Can you work these out from the model? Positions are in its coordinate system, mm. A direction names the side the tool comes from. Coordinates: 2 decimals unless noted, no trailing zeros. Loops run counter-clockwise (first coordinate to the right, second up) from the corner with the lowest first, then second, coordinate; pieces in that order, holes last. Notation, with made-up numbers: (27.5, 76) - (73.5, 76) arc R30 ccw to (73.5, 106) - close; hole circle Ø6 at (24, -22). An arc over 180 degrees is marked (long way). Put each result on its own line as item: value. Start each with the question number.
from build123d import *

# Parameters (mm, degrees)
F1_DEPTH = 800
F2_ANGLE = 180
F3_ANGLE = 270


# Not quite as in the source:
# - a feature of the source that left no trace in its solid (it failed there, or was rolled back) is left out


with BuildPart() as f1:
    # F0 (on Top) → F1 (new body)
    with BuildSketch(Plane.XY):
        Polygon((10, 0), (0, 0), (0, -10), (40, -10), (40, 30), (50, 30), (50, 80), (0, 80), (0, 70), (10, 70), (10, 72), (2.000000095, 72), (2.000000095, 78), (48, 78), (48, 32), (38, 32), (38, -8), (2, -8), (2, -2), (10, -2), align=None)
    extrude(amount=F1_DEPTH)


with BuildPart() as f1_1:
    # F2: moved
    add(f1.part.rotate(Axis((50, 55, 800), (0, 1, 0)), F2_ANGLE))


with BuildPart() as f1_2:
    # F3: moved
    add(f1_1.part.rotate(Axis((50, 55, 800), (0, 1, 0)), F3_ANGLE))


solid = f1_2.part
Q1. Please list where these lines run through material, in increasing order: line 1 along Y through (x, z) = (-266, 847.5); line 2 along Y through (x, z) = (-329.5, 809); line 3 along Y through (x, z) = (-650, 816). Write a range as [from, to].
Q2. On a 3-axis mill with a long thin cutter (end or side, diameter ignored), from which of +Z, -Z, +X, -X, +Y, -Y can I reach the whole of each face in a straight line? I mean faces 4 (the flat face through (-356, -10, 830)), 5 (the flat face through (-356, 12, 812)). Say none if no direction works.
Q3. We'd pull the mould along Y, two halves only. Please class faces 1 (the flat face through (-356, 80, 825)), 2 (the flat face through (-356, -8, 830)), 3 (the flat face through (-356, 10, 810)): released by +Y, released by -Y, zero draft, split by the parting line, or undercut.
Q4. I want a section at B-B on x = -130.5. List the corners of the cut face in (y, z) for me, and give its area (3 significant figures).
Q5. I want a section at A-A on z = 828. List the corners of the cut face in (x, y) for me.
Q6. I want a section at C-C on y = 50. List the corners of the cut face in (x, z) for me.
Q7. Will these pins go through, and if not, where does the flat tip stop? pin 1 (1 mm diameter, centred on x = -164, y = -1.5, fed in from -Z); pin 2 (1.5 mm diameter, centred on x = -77.5, y = 3, fed in from +Z).
Calculated:
1. line 1: [-10, -8], [-2, 0], [70, 72], [78, 80]
1. line 2: [30, 32], [78, 80]
1. line 3: [-10, -8], [78, 80]
2. face 4: +Z, -Z, +X, -X, -Y
2. face 5: +X, -X
3. face 1: released by +Y
3. face 2: undercut
3. face 3: zero draft
4. outline: (-10, 810) - (30, 810) - (30, 800) - (80, 800) - (80, 850) - (70, 850) - (70, 840) - (72, 840) - (72, 848) - (78, 848) - (78, 802) - (32, 802) - (32, 812) - (-8, 812) - (-8, 848) - (-2, 848) - (-2, 840) - (0, 840) - (0, 850) - (-10, 850) - close
4. area: 436 mm2
5. outline: (-750, -10) - (50, -10) - (50, -8) - (-750, -8) - close; (-750, 78) - (50, 78) - (50, 80) - (-750, 80) - close
6. outline: (-750, 800) - (50, 800) - (50, 802) - (-750, 802) - close
7. pin 1: z = 810
7. pin 2: z = 812
